Verification items for the finished model (mm, model axes). Face numbers are marked on the shaded views. A direction names the side the tool comes from. Round coordinates to 2 decimals unless told otherwise and drop trailing zeros. Order: outer loops, then holes, each group sorted by start corner. A loop starts at its lowest first (then second) coordinate and runs counter-clockwise, first axis right, second up. Notation, with made-up numbers: (-39, 81.25) -> (14, 81.25) arc R12 cw to (14, 86.25) -> close; hole circle Ø8 at (34, 54.25). An arc over 180 degrees is marked (long way). Return JSON: item names as keys, results as strings. Group by question number.
Item 1: Sectioned sample at B-B on z = -2.25. Record the cut outline in (x, y).
Item 2: Depth check by flat-ended pin: pin 1 Ø1.5 at (y, z) = (0.5, -2) entering from +X; pin 2 Ø3 at (x, z) = (0, -3.5) entering from +Y; pin 3 Ø2 at (y, z) = (0.5, -0.5) entering from +X. Enter the tip coordinate at first touch or a pass-through.
Item 3: Access from +Z, -Z, +X, -X, +Y, -Y to the whole of each face (thin tool, end or side, straight path). Record for the marked faces 4 and 5.
Item 4: Scan lines: probe 1 along Z at (x, y) = (1.5, -2); probe 2 along X at (y, z) = (0.75, -5.75); probe 3 along Z at (x, y) = (0.5, 0.75). Record each from-to range of solid material in increasing order. Write a range as from..to.
Item 5: Sectioned sample at A-A on x = 0. Record the cut outline in (y, z).
Item 6: Draft check along X on the marked faces 1, 2 and 3. Enter one of: pulls with the +X half, pulls with the -X half, needs draft (parallel to the pull), parting line crosses it, or undercut.
```python
from build123d import *

# Parameters (mm, degrees)
SKETCH_1_R          = 3
EXTRUDE_1_DEPTH     = 0.5
SKETCH_2_R          = 1.5
EXTRUDE_2_DEPTH     = 6
CHAMFER_1_SIZE      = 0.2
CUT_EXTRUDE_1_DEPTH = 0.8
FILLET_2_R          = 0.3


with BuildPart() as part:
    # 草图1 → 凸台-拉伸1 (new body, symmetric)
    with BuildSketch(Plane.XY):
        Circle(SKETCH_1_R)
    extrude(amount=EXTRUDE_1_DEPTH, both=True)

    # 草图2 → 凸台-拉伸2 (add)
    with BuildSketch(Plane(origin=(0, 0, -0.5), x_dir=(-1, 0, 0), z_dir=(0, 0, -1))):
        Circle(SKETCH_2_R)
    extrude(amount=EXTRUDE_2_DEPTH)

    # 倒角1
    chamfer_1_edges = [part.edges().sort_by_distance(p)[0] for p in [
        (1.5, 0, -6.5),
    ]]
    chamfer(chamfer_1_edges, length=CHAMFER_1_SIZE)

    # 草图3 → 切除-拉伸1 (cut)
    with BuildSketch(Plane.XY.offset(0.5)):
        Polygon((1.154700538, 0), (0.577350269, 1), (-0.577350269, 1), (-1.154700538, 0), (-0.577350269, -1), (0.577350269, -1), align=None)
    extrude(amount=-CUT_EXTRUDE_1_DEPTH, mode=Mode.SUBTRACT)

    # 圆角2
    fillet_2_edges = [part.edges().sort_by_distance(p)[0] for p in [
        (-3, 0, -0.5),
        (-3, 0, 0.5),
    ]]
    fillet(fillet_2_edges, radius=FILLET_2_R)


solid = part.part
```
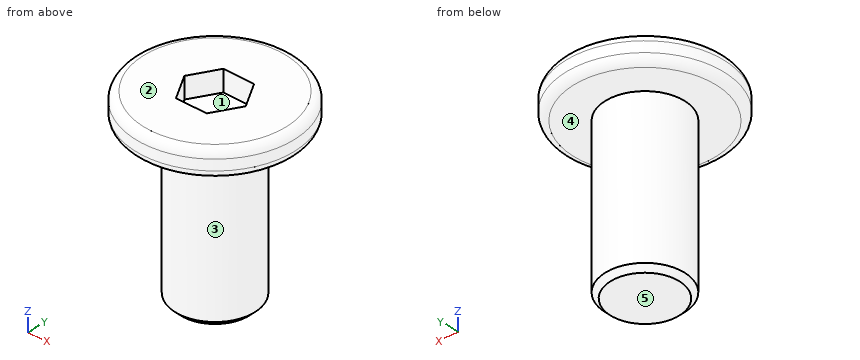
Recorded:
{
 "1": {"outline": "circle Ø3 at (0, 0)"},
 "2": {"pin 1": "x = 1.5", "pin 2": "y = 1.5", "pin 3": "x = 3"},
 "3": {"face 4": "-Z", "face 5": "-Z, +X, -X, +Y, -Y"},
 "4": {"probe 1": "-0.5..0.5", "probe 2": "-1.3..1.3", "probe 3": "-6.5..-0.3"},
 "5": {"outline": "(-3, -0.2) arc R0.3 ccw to (-2.7, -0.5) -> (-1.5, -0.5) -> (-1.5, -6.3) -> (-1.3, -6.5) -> (1.3, -6.5) -> (1.5, -6.3) -> (1.5, -0.5) -> (2.7, -0.5) arc R0.3 ccw to (3, -0.2) -> (3, 0.2) arc R0.3 ccw to (2.7, 0.5) -> (1, 0.5) -> (1, -0.3) -> (-1, -0.3) -> (-1, 0.5) -> (-2.7, 0.5) arc R0.3 ccw to (-3, 0.2) -> close"},
 "6": {"face 1": "undercut", "face 2": "needs draft", "face 3": "parting line crosses it"}
}
